Could you check a few things on this model? Use its own coordinates, in mm. A direction names the side the tool comes from. Round coordinates to 2 decimals unless told otherwise and drop trailing zeros. Write each loop counter-clockwise with the first axis right and the second up, starting at its lowest first coordinate (ties: lowest second). Pieces come first, ordered by that corner, then holes. Notation, with made-up numbers: (59.5, 77.25) - (80.5, 77.25) arc R27 cw to (80.5, 113.25) - close; hole circle Ø8 at (41.25, 22). An arc over 180 degrees is marked (long way). Put each result on its own line as item: value.
from build123d import *

# Parameters (mm, degrees)
BOSS_EXTRUDE1_DEPTH = 0.25
SKETCH2_R           = 13
BOSS_EXTRUDE2_DEPTH = 1
CIRPATTERN1_COUNT   = 3
SKETCH4_W           = 10
SKETCH4_H           = 10
BOSS_EXTRUDE3_DEPTH = 2


with BuildPart() as part:
    # Sketch1 → Boss-Extrude1 (new body, symmetric)
    with BuildSketch(Plane(origin=(0, 0, 0), x_dir=(0, 0, -1), z_dir=(1, 0, 0))):
        with BuildLine():
            Line((-1.323529412, 0.705882353), (-22.5, -39))
            Line((-22.5, -39), (22.5, -39))
            Line((22.5, -39), (1.323529412, 0.705882353))
            ThreePointArc((1.323529412, 0.705882353), (0, 1.5), (-1.323529412, 0.705882353))
        make_face()
    boss_extrude1 = extrude(amount=BOSS_EXTRUDE1_DEPTH, both=True)

    # Sketch2 → Boss-Extrude2 (add)
    with BuildSketch(Plane(origin=(0, 0, 0), x_dir=(0, 0, -1), z_dir=(1, 0, 0))):
        with Locations((0, -51.97114317)):
            Circle(SKETCH2_R)
    extrude(amount=BOSS_EXTRUDE2_DEPTH)

    # CirPattern1: Boss-Extrude1 ×3 about axis
    cirpattern1_axis = Axis((0, -51.97114317, 0), (1, 0, 0))
    for i in range(1, CIRPATTERN1_COUNT):
        add(boss_extrude1.rotate(cirpattern1_axis, i * 360 / CIRPATTERN1_COUNT))

    # Sketch4 → Boss-Extrude3 (add)
    with BuildSketch(Plane.ZY):
        with Locations((0, -51.97114317)):
            Rectangle(SKETCH4_W, SKETCH4_H)
    extrude(amount=BOSS_EXTRUDE3_DEPTH)


solid = part.part
(1) Imagine slicing it at B-B, the plane z = 18.5. List the corners of the cut face in (x, y) for me, then the cut area to 3 significant figures.
Values found:
outline: (-0.25, -78.57) - (0.25, -78.57) - (0.25, -45.87) - (-0.25, -45.87) - close; (-0.25, -39) - (0.25, -39) - (0.25, -31.5) - (-0.25, -31.5) - close
area: 20.1 mm^2
(2) I'm going to push flat-ended pins straight in: pin 1 (10 mm diameter, centred on y = -52.5, z = 26.5, fed in from -X); pin 2 (1.5 mm diameter, centred on x = 0.5, y = -70, fed in from +Z); pin 3 (1 mm diameter, centred on x = -1.5, y = -50.5, fed in from -Z). Where does each tip first touch, or does it pass through?
Values found:
pin 1: stops at x = -0.25
pin 2: stops at z = 42.26
pin 3: stops at z = -5
(3) Please list where these lines run through material, in increasing order: probe 1 along X at (y, z) = (-14, 6); probe 2 along X at (y, z) = (-50, -11.5); probe 3 along Y at (x, z) = (-1.5, -0.5). Write a range as from..to.
Values found:
probe 1: x = -0.25..0.25
probe 2: x = 0..1
probe 3: y = -56.97..-46.97
(4) For faces 4 (the face through (0, -18.86, 11.76)), 5 (the face through (0.25, -58, -12)), which set-ups out of +Z, -Z, +X, -X, +Y, -Y let a thin tool reach every point of the face, with its end or its side?
Values found:
face 4: +Z, +X, -X, +Y
face 5: +X
(5) Imagine slicing it at C-C, the plane x = -1.05. List the corners of the cut face in (y, z) for me.
Values found:
outline: (-56.97, -5) - (-46.97, -5) - (-46.97, 5) - (-56.97, 5) - close
(6) If we mould it in two halves opening along Z, with no side actions, what happens to faces 1 (the face through (0, -52, -6)), 2 (the face through (-2, -52, 0)), 3 (the face through (0.004, -19.418, -12.056))? For each: pulls with the +Z half, pulls with the -Z half, needs draft (parallel to the pull), parting line crosses it, or undercut.
Values found:
face 1: undercut
face 2: needs draft
face 3: pulls with the -Z half
(7) Imagine slicing it at D-D, the plane y = -44. List the corners of the cut face in (x, z) for me, then the cut area to 3 significant figures.
Values found:
outline: (-0.25, -25.62) - (0.25, -25.62) - (0.25, -19.58) - (-0.25, -19.58) - close; (-0.25, 19.58) - (0.25, 19.58) - (0.25, 25.62) - (-0.25, 25.62) - close; (0, -10.27) - (1, -10.27) - (1, 10.27) - (0, 10.27) - close
area: 26.6 mm^2
(8) Imagine slicing it at A-A, the plane y = -62.5. List the corners of the cut face in (x, z) for me.
Values found:
outline: (-0.25, -37.14) - (0.25, -37.14) - (0.25, -8.9) - (-0.25, -8.9) - close; (-0.25, 8.9) - (0.25, 8.9) - (0.25, 37.14) - (-0.25, 37.14) - close; (0, -7.63) - (1, -7.63) - (1, 7.63) - (0, 7.63) - close
